Design review of the part built by this model. Coordinates are the model's own, in mm. A direction names the side the tool comes from. Round coordinates to 2 decimals unless told otherwise and drop trailing zeros. Loops run counter-clockwise (first coordinate to the right, second up) from the corner with the lowest first, then second, coordinate; pieces in that order, holes last. Notation, with made-up numbers: (56.5, 26.5) - (109.5, 26.5) arc R12 ccw to (109.5, 32.5) - close; hole circle Ø7 at (60.25, 40). An arc over 180 degrees is marked (long way). Return JSON: item names as keys, results as strings. Group by question number.
(1) We need section D-D, the plane x = 37.5. Write out the cut boundary in (y, z) (3 decimals).
(2) For faces 1 (the flat face through (-3, 7.5, 2)), 2 (the flat face through (-4, -7.5, 2)), 3 (the flat face through (19, 1.588, 2)), list the 3-axis set-ups (+Z, -Z, +X, -X, +Y, -Y) from which the entire face can be reached by the end or side of a thin tool; tool diameter is ignored.
(3) We need section A-A, the plane y = 0. Write out the cut boundary in (x, z) (3 decimals), and give its area (3 significant figures).
(4) Clearance check with flat-ended pins moving along their axes: pin 1 (1 mm diameter, centred on x = 17.5, z = 1, fed in from -Y); pin 2 (1 mm diameter, centred on x = 20, z = 2, fed in from +Y); pin 3 (7.5 mm diameter, centred on x = 37.5, y = 0, fed in from -Z). State where each tip first meets the part, or that it passes through.
(5) The part is to be moulded in two halves that separate along X. For faces 4 (the cylindrical face through (-45, 0, 2)), 5 (the cylindrical face through (42.03, 1.43, 1.57)), 6 (the cylindrical face through (-34.495, 0.946, 1.565)), 7 (the flat face through (0, 0, 0)), say which applies: pulls with the +X half, pulls with the -X half, needs draft (parallel to the pull), parting line crosses it, or undercut.
(6) We need section C-C, the plane z = 1.3. Write out the cut boundary in (x, y), and give its area (3 significant figures).
(7) We need section B-B, the plane x = 22.5. Write out the cut boundary in (y, z) (1 decimal).
(8) Wall thickness on L1, parallel to Y at x = -37.5, z = 1.4; L2, parallel to X at y = 1.5, z = 1.65; L3, parallel to Y at x = 37.5, z = 1.6: over which ranges is each line inside the solid? List them lowest first. Write a range as [from, to].
from build123d import *

# Parameters (mm, degrees)
SKETCH1_R           = 3.15
SKETCH1_R_2         = 4.75
BOSS_EXTRUDE1_DEPTH = 3.175
SKETCH2_W           = 15
SKETCH2_H           = 3.175
SKETCH2_W_2         = 10
CUT_EXTRUDE1_DEPTH  = 49.349825491
SKETCH4_W           = 20.014244063
SKETCH4_H           = 7.260981568
BOSS_EXTRUDE2_DEPTH = 3.175


with BuildPart() as part:
    # Sketch1 → Boss-Extrude1 (new body)
    with BuildSketch(Plane.XY):
        with BuildLine():
            Line((-37.5, -7.5), (31.270032103, -7.5))
            ThreePointArc((31.270032103, -7.5), (47.25, 0), (31.270032103, 7.5))
            Line((31.270032103, 7.5), (-37.5, 7.5))
            ThreePointArc((-37.5, 7.5), (-45, 0), (-37.5, -7.5))
        make_face()
        with Locations((-37.5, 0)):
            Circle(SKETCH1_R, mode=Mode.SUBTRACT)
        with Locations((37.5, 0)):
            Circle(SKETCH1_R_2, mode=Mode.SUBTRACT)
    extrude(amount=BOSS_EXTRUDE1_DEPTH)

    # Sketch2 → Cut-Extrude1 (cut, through all)
    with BuildSketch(Plane.XY.offset(3.175)):
        with Locations((-17.5, 0)):
            Rectangle(SKETCH2_W, SKETCH2_H)
        with Locations((19, 0)):
            Rectangle(SKETCH2_W_2, SKETCH2_H)
    extrude(amount=-CUT_EXTRUDE1_DEPTH, mode=Mode.SUBTRACT)

    # Sketch4 → Boss-Extrude2 (add)
    with BuildSketch(Plane.XY.offset(3.175)):
        with Locations((-17.454282614, 0)):
            Rectangle(SKETCH4_W, SKETCH4_H)
    extrude(amount=-BOSS_EXTRUDE2_DEPTH)


solid = part.part
Solutions:
{
 "1": {"outline": "(-9.75, 0) - (-4.75, 0) - (-4.75, 3.175) - (-9.75, 3.175) - close; (4.75, 0) - (9.75, 0) - (9.75, 3.175) - (4.75, 3.175) - close"},
 "2": {"face 1": "+Z, -Z, -X, +Y", "face 2": "+Z, -Z, -X, -Y", "face 3": "+Z, -Z"},
 "3": {"outline": "(-45, 0) - (-40.65, 0) - (-40.65, 3.175) - (-45, 3.175) - close; (-34.35, 0) - (14, 0) - (14, 3.175) - (-34.35, 3.175) - close; (24, 0) - (32.75, 0) - (32.75, 3.175) - (24, 3.175) - close; (42.25, 0) - (47.25, 0) - (47.25, 3.175) - (42.25, 3.175) - close", "area": "211 mm^2"},
 "4": {"pin 1": "y = -7.5", "pin 2": "y = 7.5", "pin 3": "through"},
 "5": {"face 4": "pulls with the -X half", "face 5": "undercut", "face 6": "undercut", "face 7": "needs draft"},
 "6": {"outline": "(-37.5, -7.5) - (31.27, -7.5) arc R9.75 ccw (long way) to (31.27, 7.5) - (-37.5, 7.5) arc R7.5 ccw to start; hole circle Ø6.3 at (-37.5, 0); hole (14, -1.59) - (24, -1.59) - (24, 1.59) - (14, 1.59) - close; hole circle Ø9.5 at (37.5, 0)", "area": "1,250 mm^2"},
 "7": {"outline": "(-7.5, 0) - (-1.6, 0) - (-1.6, 3.2) - (-7.5, 3.2) - close; (1.6, 0) - (7.5, 0) - (7.5, 3.2) - (1.6, 3.2) - close"},
 "8": {"L1": "[-7.5, -3.15], [3.15, 7.5]", "L2": "[-44.85, -40.27], [-34.73, 14], [24, 32.99], [42.01, 47.13]", "L3": "[-9.75, -4.75], [4.75, 9.75]"}
}
